Geometry check sheet. Reference: the model listing, model coordinates, mm. A direction names the side the tool comes from. Coordinates: 2 decimals unless noted, no trailing zeros. Order: outer loops, then holes, each group sorted by start corner. A loop starts at its lowest first (then second) coordinate and runs counter-clockwise, first axis right, second up. Notation, with made-up numbers: (-28.75, 70.5) - (3.25, 70.5) arc R20 cw to (3.25, 89.5) - close; hole circle Ø2 at (-27, -26). An arc over 180 degrees is marked (long way). One line per item, written item: value. Start each with the question number.
```python
from build123d import *

# Parameters (mm, degrees)
F0_R      = 23.65
F1_DEPTH  = 25
F3_DEPTH  = 3.8
F5_DEPTH  = 15
F6_W      = 13
F6_H      = 13
F7_DEPTH  = 25.001
F8_R      = 0.15
F9_R      = 3
F10_DEPTH = 41.651


with BuildPart() as f1:
    # F0 (on Top) → F1 (new body)
    with BuildSketch(Plane.XY):
        Circle(F0_R)
    extrude(amount=F1_DEPTH)

    # F2 (on face) → F3 (cut)
    with BuildSketch(Plane(origin=(0, 0, 0), x_dir=(1, 0, 0), z_dir=(0, 0, -1))):
        with BuildLine():
            Line((-2, 20.954773), (-2, 23.565282))
            ThreePointArc((-2, 23.565282), (-9.050463, 21.849751), (-15.248957, 18.077384))
            Line((-15.248957, 18.077384), (-13.403048, 16.231475))
            ThreePointArc((-13.403048, 16.231475), (-8.055486, 19.447664), (-2, 20.954773))
        make_face()
        with BuildLine():
            ThreePointArc((21.05, 0), (21.02618, 1.001133), (20.954773, 2))
            ThreePointArc((20.954773, 2), (19.447664, 8.055486), (16.231475, 13.403048))
            ThreePointArc((16.231475, 13.403048), (14.884598, 14.884598), (13.403048, 16.231475))
            ThreePointArc((13.403048, 16.231475), (8.055486, 19.447664), (2, 20.954773))
            ThreePointArc((2, 20.954773), (0, 21.05), (-2, 20.954773))
            ThreePointArc((-2, 20.954773), (-8.055486, 19.447664), (-13.403048, 16.231475))
            ThreePointArc((-13.403048, 16.231475), (-14.884598, 14.884598), (-16.231475, 13.403048))
            ThreePointArc((-16.231475, 13.403048), (-19.447664, 8.055486), (-20.954773, 2))
            ThreePointArc((-20.954773, 2), (-21.05, 0), (-20.954773, -2))
            ThreePointArc((-20.954773, -2), (-19.447664, -8.055486), (-16.231475, -13.403048))
            ThreePointArc((-16.231475, -13.403048), (-14.884598, -14.884598), (-13.403048, -16.231475))
            ThreePointArc((-13.403048, -16.231475), (-8.055486, -19.447664), (-2, -20.954773))
            ThreePointArc((-2, -20.954773), (0, -21.05), (2, -20.954773))
            ThreePointArc((2, -20.954773), (8.055486, -19.447664), (13.403048, -16.231475))
            ThreePointArc((13.403048, -16.231475), (14.884598, -14.884598), (16.231475, -13.403048))
            ThreePointArc((16.231475, -13.403048), (19.447664, -8.055486), (20.954773, -2))
            ThreePointArc((20.954773, -2), (21.02618, -1.001133), (21.05, 0))
        make_face()
        with BuildLine():
            Line((-16.231475, 13.403048), (-18.077384, 15.248957))
            ThreePointArc((-18.077384, 15.248957), (-21.849751, 9.050463), (-23.565282, 2))
            Line((-23.565282, 2), (-20.954773, 2))
            ThreePointArc((-20.954773, 2), (-19.447664, 8.055486), (-16.231475, 13.403048))
        make_face()
        with BuildLine():
            ThreePointArc((-23.565282, -2), (-21.849751, -9.050463), (-18.077384, -15.248957))
            Line((-18.077384, -15.248957), (-16.231475, -13.403048))
            ThreePointArc((-16.231475, -13.403048), (-19.447664, -8.055486), (-20.954773, -2))
            Line((-20.954773, -2), (-23.565282, -2))
        make_face()
        with BuildLine():
            ThreePointArc((-15.248957, -18.077384), (-9.050463, -21.849751), (-2, -23.565282))
            Line((-2, -23.565282), (-2, -20.954773))
            ThreePointArc((-2, -20.954773), (-8.055486, -19.447664), (-13.403048, -16.231475))
            Line((-13.403048, -16.231475), (-15.248957, -18.077384))
        make_face()
        with BuildLine():
            ThreePointArc((2, -23.565282), (9.050463, -21.849751), (15.248957, -18.077384))
            Line((15.248957, -18.077384), (13.403048, -16.231475))
            ThreePointArc((13.403048, -16.231475), (8.055486, -19.447664), (2, -20.954773))
            Line((2, -20.954773), (2, -23.565282))
        make_face()
        with BuildLine():
            ThreePointArc((18.077384, -15.248957), (21.849751, -9.050463), (23.565282, -2))
            Line((23.565282, -2), (20.954773, -2))
            ThreePointArc((20.954773, -2), (19.447664, -8.055486), (16.231475, -13.403048))
            Line((16.231475, -13.403048), (18.077384, -15.248957))
        make_face()
        with BuildLine():
            Line((20.954773, 2), (23.565282, 2))
            ThreePointArc((23.565282, 2), (21.849751, 9.050463), (18.077384, 15.248957))
            Line((18.077384, 15.248957), (16.231475, 13.403048))
            ThreePointArc((16.231475, 13.403048), (19.447664, 8.055486), (20.954773, 2))
        make_face()
        with BuildLine():
            Line((13.403048, 16.231475), (15.248957, 18.077384))
            ThreePointArc((15.248957, 18.077384), (9.050463, 21.849751), (2, 23.565282))
            Line((2, 23.565282), (2, 20.954773))
            ThreePointArc((2, 20.954773), (8.055486, 19.447664), (13.403048, 16.231475))
        make_face()
    extrude(amount=-F3_DEPTH, mode=Mode.SUBTRACT)

    # F4 (on face) → F5 (cut)
    with BuildSketch(Plane.XY.offset(25)):
        with BuildLine():
            Line((-18, -15.340225), (-18, 15.340225))
            ThreePointArc((-18, 15.340225), (-23.65, 0), (-18, -15.340225))
        make_face()
        with BuildLine():
            Line((18, 15.340225), (18, -15.340225))
            ThreePointArc((18, -15.340225), (23.65, 0), (18, 15.340225))
        make_face()
    extrude(amount=-F5_DEPTH, mode=Mode.SUBTRACT)

    # F6 (on face) → F7 (cut, through all)
    with BuildSketch(Plane.XY.offset(25)):
        Rectangle(F6_W, F6_H)
    extrude(amount=-F7_DEPTH, mode=Mode.SUBTRACT)

    # F8
    f8_edges = [f1.edges().sort_by_distance(p)[0] for p in [
        (-6.5, 6.5, 14.4),
        (-6.5, -6.5, 14.4),
        (6.5, 6.5, 14.4),
        (6.5, -6.5, 14.4),
    ]]
    fillet(f8_edges, radius=F8_R)

    # F9 (on face) → F10 (cut, through all)
    with BuildSketch(Plane.YZ.offset(18)):
        with Locations((0, 17)):
            Circle(F9_R)
    extrude(amount=-F10_DEPTH, mode=Mode.SUBTRACT)


solid = f1.part
```
Q1. Cross-section at A-A, the plane x = 0. Enter the section's corners in (y, z).
Q2. Cross-section at D-D, the plane y = -10. Enter the section's corners in (x, z), and give its area (3 significant figures).
Q3. Cross-section at C-C, the plane z = 11.75. Enter the section's corners in (x, y).
Q4. Set-up check for faces 4 (the flat face through (22, 2, 2)), 5 (the cylindrical face through (0.03, -21.05, 1.87)), 6 (the flat face through (6.5, 0, 12)), 7 (the flat face through (14.34, 17.17, 1.87)): record each of +Z, -Z, +X, -X, +Y, -Y from which the full face is reachable in a straight line by a thin tool's end or side.
Q5. Release check for a two-part mould opening along Y. For faces 1 (the flat face through (-14.31, 17.14, 1.87)), 2 (the flat face through (-18, 0, 21)), 3 (the flat face through (0, -6.5, 15)) record: released by +Y, released by -Y, zero draft, split by the parting line, or undercut.
Q6. Gauge pin test, flat ends, axial feed: P1, Ø3, axis at y = 22, z = 2, coming from the -X side; P2, Ø6, axis at x = 3.5, z = 14, coming from the +Y side; P3, Ø9.5, axis at y = 0, z = 17, coming from the +X side. Record the tip position at first contact, or that the pin passes through.
Q7. Material ranges on probe 1 along Z at (x, y) = (11.25, 0); probe 2 along Z at (x, y) = (19.5, -4.5); probe 3 along X at (y, z) = (-7.5, 19.5), recorded low to high.
Q8. Cross-section at B-B, the plane z = 17. Enter the section's corners in (x, y).
Check result:
1. outline: (-23.65, 0) - (-21.05, 0) - (-21.05, 3.8) - (-6.5, 3.8) - (-6.5, 25) - (-23.65, 25) - close; (6.5, 3.8) - (21.05, 3.8) - (21.05, 0) - (23.65, 0) - (23.65, 25) - (6.5, 25) - close
2. outline: (-21.43, 3.8) - (21.43, 3.8) - (21.43, 10) - (18, 10) - (18, 25) - (-18, 25) - (-18, 10) - (-21.43, 10) - close
2. area: 806 mm2
3. outline: (-18, -15.34) arc R23.65 ccw to (18, -15.34) - (18, 15.34) arc R23.65 ccw to (-18, 15.34) - close; hole (-6.5, -6.35) arc R0.15 ccw to (-6.35, -6.5) - (6.35, -6.5) arc R0.15 ccw to (6.5, -6.35) - (6.5, 6.35) arc R0.15 ccw to (6.35, 6.5) - (-6.35, 6.5) arc R0.15 ccw to (-6.5, 6.35) - close
4. face 4: -Z, +X, -X, +Y
4. face 5: -Z
4. face 6: +Z, -Z
4. face 7: -Z, +Y
5. face 1: released by +Y
5. face 2: zero draft
5. face 3: undercut
6. P1: stops at x = -2
6. P2: stops at y = 23.64
6. P3: stops at x = 18
7. probe 1: z = 3.8 to 14, 20 to 25
7. probe 2: z = 3.8 to 10
7. probe 3: x = -18 to 18
8. outline: (-18, -15.34) arc R23.65 ccw to (18, -15.34) - (18, -3) - (6.5, -3) - (6.5, -6.35) arc R0.15 cw to (6.35, -6.5) - (-6.35, -6.5) arc R0.15 cw to (-6.5, -6.35) - (-6.5, -3) - (-18, -3) - close; (-18, 3) - (-6.5, 3) - (-6.5, 6.35) arc R0.15 cw to (-6.35, 6.5) - (6.35, 6.5) arc R0.15 cw to (6.5, 6.35) - (6.5, 3) - (18, 3) - (18, 15.34) arc R23.65 ccw to (-18, 15.34) - close
